from build123d import *

# Parameters (mm, degrees)
EXTRUDE1_DEPTH = 1.5


with BuildPart() as part:
    # Sketch1 → Extrude1 (new body)
    with BuildSketch(Plane.XY):
        with BuildLine():
            Line((70.775, 15.7), (72.275, 15.7))
            Line((72.275, 15.7), (72.275, 2.5))
            Line((72.275, 2.5), (70.125, 2.5))
            Line((70.125, 2.5), (70.125, 0))
            Line((70.125, 0), (53.775, 0))
            Line((53.775, 0), (53.775, 2.5))
            Line((53.775, 2.5), (51.625, 2.5))
            Line((51.625, 2.5), (49.475, 2.5))
            Line((49.475, 2.5), (49.475, 0))
            Line((49.475, 0), (33.125, 0))
            Line((33.125, 0), (33.125, 2.5))
            Line((33.125, 2.5), (30.975, 2.5))
            Line((30.975, 2.5), (28.825, 2.5))
            Line((28.825, 2.5), (28.825, 0))
            Line((28.825, 0), (12.475, 0))
            Line((12.475, 0), (12.475, 2.5))
            Line((12.475, 2.5), (10.325, 2.5))
            Line((10.325, 2.5), (8.175, 2.5))
            Line((8.175, 2.5), (8.175, 0))
            Line((8.175, 0), (-8.175, 0))
            Line((-8.175, 0), (-8.175, 2.5))
            Line((-8.175, 2.5), (-10.325, 2.5))
            Line((-10.325, 2.5), (-10.325, 15.7))
            Line((-10.325, 15.7), (-8.825000006, 15.7))
            add(Edge.make_bspline(
                [(-8.825000006, 15.7), (-5.625000003, 19.70356859), (-2.425, 14.6)],
                knots=[0, 0, 0, 1, 1, 1], degree=2))
            Line((-2.425, 14.6), (2.425000009, 14.6))
            add(Edge.make_bspline(
                [(2.425000009, 14.6), (5.625000004, 19.703568583), (8.825, 15.7)],
                knots=[0, 0, 0, 1, 1, 1], degree=2))
            Line((8.825, 15.7), (10.325, 15.7))
            Line((10.325, 15.7), (11.824999994, 15.7))
            add(Edge.make_bspline(
                [(11.824999994, 15.7), (15.024999997, 19.70356859), (18.225, 14.6)],
                knots=[0, 0, 0, 1, 1, 1], degree=2))
            Line((18.225, 14.6), (23.075000009, 14.6))
            add(Edge.make_bspline(
                [(23.075000009, 14.6), (26.275000004, 19.703568583), (29.475, 15.7)],
                knots=[0, 0, 0, 1, 1, 1], degree=2))
            Line((29.475, 15.7), (30.975, 15.7))
            Line((30.975, 15.7), (32.474999994, 15.7))
            add(Edge.make_bspline(
                [(32.474999994, 15.7), (35.674999997, 19.70356859), (38.875, 14.6)],
                knots=[0, 0, 0, 1, 1, 1], degree=2))
            Line((38.875, 14.6), (43.725000009, 14.6))
            add(Edge.make_bspline(
                [(43.725000009, 14.6), (46.925000004, 19.703568583), (50.125, 15.7)],
                knots=[0, 0, 0, 1, 1, 1], degree=2))
            Line((50.125, 15.7), (51.625, 15.7))
            Line((51.625, 15.7), (53.124999994, 15.7))
            add(Edge.make_bspline(
                [(53.124999994, 15.7), (56.324999997, 19.70356859), (59.525, 14.6)],
                knots=[0, 0, 0, 1, 1, 1], degree=2))
            Line((59.525, 14.6), (64.375000009, 14.6))
            add(Edge.make_bspline(
                [(64.375000009, 14.6), (67.575000004, 19.703568583), (70.775, 15.7)],
                knots=[0, 0, 0, 1, 1, 1], degree=2))
        make_face()
    extrude(amount=EXTRUDE1_DEPTH)


solid = part.part
Model file for the job. Use its own axes, mm. A direction names the side the tool comes from. Round coordinates to 2 decimals unless told otherwise and drop trailing zeros. Loops run counter-clockwise (first coordinate to the right, second up) from the corner with the lowest first, then second, coordinate; pieces in that order, holes last. Notation, with made-up numbers: (42.5, 33.25) - (97.5, 33.25) arc R19 cw to (97.5, 38.25) - close; hole circle Ø9 at (10, 21.25). An arc over 180 degrees is marked (long way). Write each question's results on one line, items separated by ' | '.
(1) Mould opens along X. For faces 1 (the flat face through (12.475, 1, 1)), 2 (the flat face through (62, 0, 1)), 3 (the flat face through (70.125, 1, 1)) say: released by +X, released by -X, zero draft, split by the parting line, or undercut.
Answer below:
face 1: undercut | face 2: zero draft | face 3: released by +X
(2) Saw through at A-A, the plane x = -1. List the corners of the cut face in (y, z).
Answer below:
outline: (0, 0) - (14.6, 0) - (14.6, 1.5) - (0, 1.5) - close
(3) Wall check: L1, parallel to X at y = 2, z = 0.3 (3 decimals); L2, parallel to Y at x = 1, z = 0.8; L3, parallel to Y at x = 52.5, z = 1.4. Give the ranges that are in metal, low to high.
Answer below:
L1: x = -8.175 to 8.175, 12.475 to 28.825, 33.125 to 49.475, 53.775 to 70.125 | L2: y = 0 to 14.6 | L3: y = 2.5 to 15.7
(4) 3-axis set-ups, long thin cutter, end or side, ignore diameter. For faces 4 (the flat face through (0, 14.6, 1)), 5 (the flat face through (-8.175, 1, 1)), 6 (the flat face through (72, 15.7, 1)), 7 (the flat face through (33.125, 1, 1)): which of +Z, -Z, +X, -X, +Y, -Y reach the whole face in a straight line?
Answer below:
face 4: +Z, -Z, +Y | face 5: +Z, -Z, -X, -Y | face 6: +Z, -Z, +X, +Y | face 7: +Z, -Z, -Y
(5) Pin check, flat tips, straight feed: pin 1 (0.8 mm diameter, centred on x = -9.5, z = 0.5, fed in from -Y); pin 2 (0.8 mm diameter, centred on y = 0.5, z = 0.5, fed in from -X) (3 decimals). Stop position of each tip, or through.
Answer below:
pin 1: stops at y = 2.5 | pin 2: stops at x = -8.175
